CAD build for the part. Positions are in the model's coordinates, mm. A direction names the side the tool comes from. Round coordinates to 2 decimals unless told otherwise and drop trailing zeros. Loops run counter-clockwise (first coordinate to the right, second up) from the corner with the lowest first, then second, coordinate; pieces in that order, holes last.
```python
from build123d import *

# Parameters (mm, degrees)
EXTRUDE_1_DEPTH             = 24
EXTRUDE_1_DEPTH_BACK        = 6
EXTRUDE_2_DEPTH             = 18
HOLE_WIZARD_M61_D           = 6.6
HOLE_WIZARD_M61_CBORE_D     = 11
HOLE_WIZARD_M61_CBORE_DEPTH = 6.4


with BuildPart() as part:
    # Эскиз1 → Бобышка-Вытянуть1 (new, two sides: drawn at the far end of the back side and taken through both)
    with BuildSketch(Plane.XY.offset(-EXTRUDE_1_DEPTH_BACK)):
        with BuildLine():
            Line((28.5, 12), (40, 12))
            Line((40, 12), (40, 0))
            Line((40, 0), (0, 0))
            Line((0, 0), (0, 12))
            Line((0, 12), (11.5, 12))
            ThreePointArc((11.5, 12), (20, 3.5), (28.5, 12))
        make_face()
    extrude(amount=EXTRUDE_1_DEPTH + EXTRUDE_1_DEPTH_BACK)

    # Эскиз3 → Бобышка-Вытянуть2 (add)
    with BuildSketch(Plane.XY):
        with BuildLine():
            Line((11.5, 12), (14, 12))
            ThreePointArc((14, 12), (20, 6), (26, 12))
            Line((26, 12), (28.5, 12))
            ThreePointArc((28.5, 12), (20, 3.5), (11.5, 12))
        make_face()
    extrude(amount=EXTRUDE_2_DEPTH)

    # Цековка для  винта с внутренним шестигранником M61 (through all)
    with Locations(Plane.XZ):
        with Locations((7.5, 9), (32.5, 9)):
            CounterBoreHole(HOLE_WIZARD_M61_D / 2, HOLE_WIZARD_M61_CBORE_D / 2, HOLE_WIZARD_M61_CBORE_DEPTH)


solid = part.part
```
Item 1: Cut at A-A, the plane x = 32.5. Give the cut face in (y, z).
Answers follow:
outline: (0, -6) - (12, -6) - (12, 5.7) - (6.4, 5.7) - (6.4, 3.5) - (0, 3.5) - close; (0, 14.5) - (6.4, 14.5) - (6.4, 12.3) - (12, 12.3) - (12, 24) - (0, 24) - close
Item 2: Cut at C-C, the plane z = 9. Give the cut face in (x, y).
Answers follow:
outline: (0, 0) - (2, 0) - (2, 6.4) - (4.2, 6.4) - (4.2, 12) - (0, 12) - close; (10.8, 6.4) - (13, 6.4) - (13, 0) - (27, 0) - (27, 6.4) - (29.2, 6.4) - (29.2, 12) - (26, 12) arc R6 cw to (14, 12) - (10.8, 12) - close; (35.8, 6.4) - (38, 6.4) - (38, 0) - (40, 0) - (40, 12) - (35.8, 12) - close
Item 3: Two-plate mould, pull along X, no slides. Class faces 1 (the flat face through (36, 6.4, 9)), 2 (the flat face through (40, 6, 9)), 3 (the flat face through (20, 0, 9)): released by +X, released by -X, zero draft, split by the parting line, or undercut.
Answers follow:
face 1: undercut
face 2: released by +X
face 3: zero draft
Item 4: Flat gauge pins, fed straight in: P1, Ø2.5, axis at x = 22.5, y = 7, coming from the +Z side; P2, Ø10.5, axis at x = 7.5, z = 9, coming from the -Y side. Where does each tip first touch, or does it go through?
Answers follow:
P1: stops at z = 18
P2: stops at y = 6.4
Item 5: Cut at D-D, the plane x = 20. Give the cut face in (y, z), plus the area to 3 significant figures.
Answers follow:
outline: (0, -6) - (3.5, -6) - (3.5, 0) - (6, 0) - (6, 18) - (3.5, 18) - (3.5, 24) - (0, 24) - close
area: 150 mm2
Item 6: 3-axis set-ups, long thin cutter, end or side, ignore diameter. For faces 4 (the flat face through (20, 5, 18)), 5 (the cylindrical face through (19.813, 3.502, -3.042)), 6 (the flat face through (11, 6.4, 9)), 7 (the flat face through (4, 12, 9)): which of +Z, -Z, +X, -X, +Y, -Y reach the whole face in a straight line?
Answers follow:
face 4: +Z, +Y
face 5: -Z, +Y
face 6: -Y
face 7: +Z, -Z, +X, -X, +Y
Item 7: Probe line 1 (Z direction, x = 7.5, y = 5); line 2 (Z direction, x = 7.5, y = 9.45); line 3 (X direction, y = 8, z = 8.25). List the from-to ranges inside material, lowest first.
Answers follow:
line 1: z = -6 to 3.5, 14.5 to 24
line 2: z = -6 to 5.7, 12.3 to 24
line 3: x = 0 to 4.29, 10.71 to 15.53, 24.47 to 29.29, 35.71 to 40
Item 8: Cut at B-B, the plane y = 9.5. Give the cut face in (x, z), plus the area to 3 significant figures.
Answers follow:
outline: (0, -6) - (11.88, -6) - (11.88, 0) - (14.55, 0) - (14.55, 18) - (11.88, 18) - (11.88, 24) - (0, 24) - close; (25.45, 0) - (28.12, 0) - (28.12, -6) - (40, -6) - (40, 24) - (28.12, 24) - (28.12, 18) - (25.45, 18) - close; hole circle Ø6.6 at (7.5, 9); hole circle Ø6.6 at (32.5, 9)
area: 740 mm2
